Read the model definition and answer for the solid it produces. Units are mm, in the model's axes. A direction names the side the tool comes from. Coordinates: 2 decimals unless noted, no trailing zeros. Write each loop counter-clockwise with the first axis right and the second up, starting at its lowest first coordinate (ties: lowest second). Pieces come first, ordered by that corner, then holes.
(1) Determine the mould class of faces 4 (the flat face through (-69.5, -7, -104)), 5 (the flat face through (-35.5, -7, -106)), 6 (the conical face through (-83.538, 0.703, -86.907)) for opening direction X: pulls with the +X half, pulls with the -X half, needs draft (parallel to the pull), parting line crosses it, or undercut.
(2) The part is cut by section B-B, the plane x = 14. Determine the outline of the cut face in (y, z), and give its area (3 significant figures).
(3) Which of the six approach directions +Z, -Z, +X, -X, +Y, -Y give full straight-line access (tool end or side, diameter ignored) to faces 1 (the flat face through (-65, -7, -109.5)), 2 (the flat face through (-59.5, -7, -104)), 3 (the flat face through (-44, -7, -115.5))?
(4) The part is cut by section C-C, the plane z = 40. Determine the outline of the cut face in (x, y), and give its area (3 significant figures).
(5) The part is cut by section A-A, the plane y = -12.25. Determine the outline of the cut face in (x, z), and give its area (3 significant figures).
(6) Given pin 1 (5 mm diameter, centred on x = -62.5, y = -9.5, fed in from -Z); pin 2 (6 mm diameter, centred on y = -6.5, z = -100.5, fed in from -X); pin 3 (7.5 mm diameter, centred on y = -6.5, z = -103, fed in from +X); pin 4 (2.5 mm diameter, centred on x = -85, z = 85, fed in from +Y), each flat-ended and moving along its own axis, determine where each tip first touches the part or whether it passes through.
(7) Straight lines are drawn through the part: line 1 along X through (y, z) = (0.35, -85); line 2 along X through (y, z) = (-2.25, -101.5). For each, find the intervals that lie inside material, in ascending order.
```python
from build123d import *

# Parameters (mm, degrees)
SKETCH1_W                                      = 235
SKETCH1_H                                      = 235
BOSS_EXTRUDE1_DEPTH                            = 3
CSK_FOR_M4_FLAT_HEAD_MACHINE_SCREW1_AT_2_COUNT = 2
CSK_FOR_M4_FLAT_HEAD_MACHINE_SCREW1_AT_2_PITCH = 170
CSK_FOR_M4_FLAT_HEAD_MACHINE_SCREW1_AT_3_COUNT = 2
CSK_FOR_M4_FLAT_HEAD_MACHINE_SCREW1_AT_3_PITCH = 240.416305603
CSK_FOR_M4_FLAT_HEAD_MACHINE_SCREW1_AT_4_COUNT = 2
CSK_FOR_M4_FLAT_HEAD_MACHINE_SCREW1_AT_4_PITCH = 170
SKETCH9_W                                      = 10
SKETCH9_H                                      = 12
SKETCH9_W_2                                    = 17
SKETCH9_H_2                                    = 20
BOSS_EXTRUDE5_DEPTH                            = 15


with BuildPart() as part:
    # Sketch1 → Boss-Extrude1 (new body)
    with BuildSketch(Plane(origin=(0, 0, 0), x_dir=(1, 0, 0), z_dir=(0, 1, 0))):
        Rectangle(SKETCH1_W, SKETCH1_H)
    extrude(amount=BOSS_EXTRUDE1_DEPTH)

    # Sketch3 → CSK for M4 Flat Head Machine Screw1 (revolve, cut)
    with BuildSketch(Plane(origin=(-85, 3, -85), x_dir=(0, 0, 1), z_dir=(1, 0, 0))):
        Polygon((0, 0), (0, 3), (2.25, 3), (2.25, 2.45), (4.7, 0), align=None)
    csk_for_m4_flat_head_machine_screw1 = revolve(axis=Axis((-85, 9.35, -85), (0, -1, 0)), mode=Mode.SUBTRACT)

    # CSK for M4 Flat Head Machine Screw1 at 2: CSK for M4 Flat Head Machine Screw1 ×2
    with Locations(*[(i * CSK_FOR_M4_FLAT_HEAD_MACHINE_SCREW1_AT_2_PITCH, 0, 0) for i in range(1, CSK_FOR_M4_FLAT_HEAD_MACHINE_SCREW1_AT_2_COUNT)]):
        add(csk_for_m4_flat_head_machine_screw1, mode=Mode.SUBTRACT)

    # CSK for M4 Flat Head Machine Screw1 at 3: CSK for M4 Flat Head Machine Screw1 ×2
    with Locations(*[Vector(0.707106781, 0, 0.707106781) * (i * CSK_FOR_M4_FLAT_HEAD_MACHINE_SCREW1_AT_3_PITCH) for i in range(1, CSK_FOR_M4_FLAT_HEAD_MACHINE_SCREW1_AT_3_COUNT)]):
        add(csk_for_m4_flat_head_machine_screw1, mode=Mode.SUBTRACT)

    # CSK for M4 Flat Head Machine Screw1 at 4: CSK for M4 Flat Head Machine Screw1 ×2
    with Locations(*[(0, 0, i * CSK_FOR_M4_FLAT_HEAD_MACHINE_SCREW1_AT_4_PITCH) for i in range(1, CSK_FOR_M4_FLAT_HEAD_MACHINE_SCREW1_AT_4_COUNT)]):
        add(csk_for_m4_flat_head_machine_screw1, mode=Mode.SUBTRACT)

    # Sketch9 → Boss-Extrude5 (add)
    with BuildSketch(Plane.XZ):
        with Locations((-64.5, -103.5)):
            Rectangle(SKETCH9_W, SKETCH9_H)
        with Locations((-44, -105.5)):
            Rectangle(SKETCH9_W_2, SKETCH9_H_2)
    extrude(amount=BOSS_EXTRUDE5_DEPTH)


solid = part.part
```
Computed:
1. face 4: pulls with the -X half
1. face 5: pulls with the +X half
1. face 6: undercut
2. outline: (0, -117.5) - (3, -117.5) - (3, 117.5) - (0, 117.5) - close
2. area: 705 mm2
3. face 1: -Z, -X, -Y
3. face 2: +Z, -Z, -Y
3. face 3: -Z, +X, -X, -Y
4. outline: (-117.5, 0) - (117.5, 0) - (117.5, 3) - (-117.5, 3) - close
4. area: 705 mm2
5. outline: (-69.5, -109.5) - (-59.5, -109.5) - (-59.5, -97.5) - (-69.5, -97.5) - close; (-52.5, -115.5) - (-35.5, -115.5) - (-35.5, -95.5) - (-52.5, -95.5) - close
5. area: 460 mm2
6. pin 1: stops at z = -109.5
6. pin 2: stops at x = -69.5
6. pin 3: stops at x = -35.5
6. pin 4: passes through
7. line 1: x = -117.5 to -87.25, -82.75 to 82.75, 87.25 to 117.5
7. line 2: x = -69.5 to -59.5, -52.5 to -35.5
